Verification items for the finished model (mm, model axes). Face numbers are marked on the shaded views. A direction names the side the tool comes from. Coordinates: 2 decimals unless noted, no trailing zeros. Loops run counter-clockwise (first coordinate to the right, second up) from the corner with the lowest first, then second, coordinate; pieces in that order, holes last. Notation, with made-up numbers: (39.5, 85) -> (78.5, 85) arc R26 cw to (78.5, 108) -> close; hole circle Ø7 at (57.25, 61.25). An arc over 180 degrees is marked (long way). Write item = value, one per line.
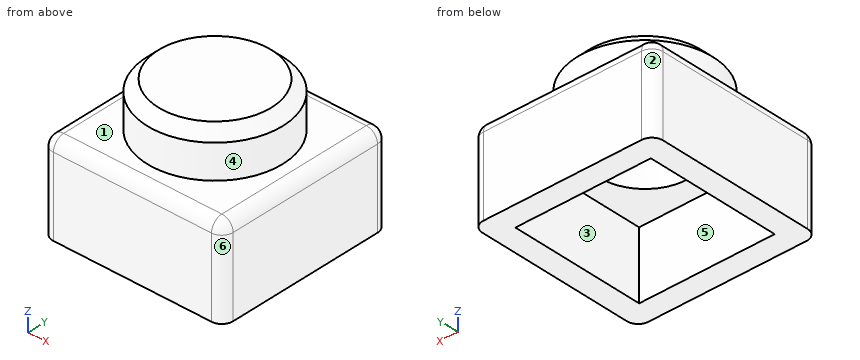
```python
from build123d import *

# Parameters (mm, degrees)
SKETCH_1_W          = 80
SKETCH_1_H          = 80
EXTRUDE_1_DEPTH     = 40
SKETCH_2_R          = 30
EXTRUDE_2_DEPTH     = 20
SKETCH_3_W          = 60
SKETCH_3_H          = 60
CUT_EXTRUDE_1_DEPTH = 30
SKETCH_4_R          = 20
CUT_EXTRUDE_2_DEPTH = 20
CHAMFER_1_SIZE      = 5
FILLET_1_R          = 5


with BuildPart() as part:
    # 草图1 → 凸台-拉伸1 (new body)
    with BuildSketch(Plane.XY):
        Rectangle(SKETCH_1_W, SKETCH_1_H)
    extrude(amount=EXTRUDE_1_DEPTH)

    # 草图2 → 凸台-拉伸2 (add)
    with BuildSketch(Plane.XY.offset(40)):
        Circle(SKETCH_2_R)
    extrude(amount=EXTRUDE_2_DEPTH)

    # 草图3 → 切除-拉伸1 (cut)
    with BuildSketch(Plane(origin=(0, 0, 0), x_dir=(-1, 0, 0), z_dir=(0, 0, -1))):
        Rectangle(SKETCH_3_W, SKETCH_3_H)
    extrude(amount=-CUT_EXTRUDE_1_DEPTH, mode=Mode.SUBTRACT)

    # 草图4 → 切除-拉伸2 (cut)
    with BuildSketch(Plane(origin=(0, 0, 30), x_dir=(-1, 0, 0), z_dir=(0, 0, -1))):
        Circle(SKETCH_4_R)
    extrude(amount=-CUT_EXTRUDE_2_DEPTH, mode=Mode.SUBTRACT)

    # 倒角1
    chamfer_1_edges = [part.edges().sort_by_distance(p)[0] for p in [
        (-30, 0, 60),
    ]]
    chamfer(chamfer_1_edges, length=CHAMFER_1_SIZE)

    # 圆角1
    fillet_1_edges = [part.edges().sort_by_distance(p)[0] for p in [
        (-40, 0, 40),
        (0, -40, 40),
        (40, 0, 40),
        (40, -40, 20),
        (-40, -40, 20),
        (-40, 40, 20),
        (40, 40, 20),
        (0, 40, 40),
    ]]
    fillet(fillet_1_edges, radius=FILLET_1_R)


solid = part.part
```
1) Sectioned sample at D-D, the plane z = 13.5. Record the cut outline in (x, y), plus the area to 3 significant figures.
Ans:
outline = (-40, -35) arc R5 ccw to (-35, -40) -> (35, -40) arc R5 ccw to (40, -35) -> (40, 35) arc R5 ccw to (35, 40) -> (-35, 40) arc R5 ccw to (-40, 35) -> close; hole (-30, -30) -> (30, -30) -> (30, 30) -> (-30, 30) -> close
area = 2,780 mm2
2) Sectioned sample at A-A, the plane z = 33. Record the cut outline in (x, y), plus the area to 3 significant figures.
Ans:
outline = (-40, -35) arc R5 ccw to (-35, -40) -> (35, -40) arc R5 ccw to (40, -35) -> (40, 35) arc R5 ccw to (35, 40) -> (-35, 40) arc R5 ccw to (-40, 35) -> close; hole circle Ø40 at (0, 0)
area = 5,120 mm2
3) Release check for a two-part mould opening along Y. For the marked faces 1, 2 and 3 record: pulls with the +Y half, pulls with the -Y half, needs draft (parallel to the pull), parting line crosses it, or undercut.
Ans:
face_1 = needs draft
face_2 = pulls with the +Y half
face_3 = undercut
4) Material ranges on line 1 (Y direction, x = 0, z = 43); line 2 (Y direction, x = -1, z = 27.5), recorded low to high.
Ans:
line_1 = -30 to -20, 20 to 30
line_2 = -40 to -30, 30 to 40
5) Sectioned sample at B-B, the plane y = 0. Record the cut outline in (x, z).
Ans:
outline = (-40, 0) -> (-30, 0) -> (-30, 30) -> (-20, 30) -> (-20, 50) -> (20, 50) -> (20, 30) -> (30, 30) -> (30, 0) -> (40, 0) -> (40, 35) arc R5 ccw to (35, 40) -> (30, 40) -> (30, 55) -> (25, 60) -> (-25, 60) -> (-30, 55) -> (-30, 40) -> (-35, 40) arc R5 ccw to (-40, 35) -> close
6) Depth check by flat-ended pin: pin 1 Ø10 at (x, z) = (-12, 45.5) entering from -Y; pin 2 Ø2 at (y, z) = (12, 45) entering from -X; pin 3 Ø5 at (y, z) = (5, 41.5) entering from +X. Enter the tip coordinate at first touch or a pass-through.
Ans:
pin_1 = -29.17
pin_2 = -27.91
pin_3 = 38
7) Tool access check on the marked faces 4, 5 and 6. Record the directions out of +Z, -Z, +X, -X, +Y, -Y that give a thin tool (end or side, any length) a straight path to the whole face; none if there is none.
Ans:
face_4 = +Z
face_5 = -Z
face_6 = +Z, -Z, +X, -Y
